Here's how the part is built. I have some questions about the finished solid (model axes, mm). A direction names the side the tool comes from. Round coordinates to 2 decimals unless told otherwise and drop trailing zeros. Write each loop counter-clockwise with the first axis right and the second up, starting at its lowest first coordinate (ties: lowest second). Pieces come first, ordered by that corner, then holes. Notation, with made-up numbers: (29.5, -0.5) - (66.5, -0.5) arc R8 ccw to (66.5, 11.5) - close; hole circle Ø6 at (-2, 66). An arc over 180 degrees is marked (long way). Return JSON: item names as keys, results as strings. Group by question number.
```python
from build123d import *

# Parameters (mm, degrees)
F0_W     = 48.26
F0_H     = 23.622
F1_DEPTH = 1.5875
F2_R     = 2.794
F2_R_2   = 1.016
F3_DEPTH = 3.175
F4_DEPTH = 6.35
F5_W     = 7.62
F5_H     = 12.7
F6_DEPTH = 6.35


with BuildPart() as f1:
    # F0 (on Top) → F1 (new body)
    with BuildSketch(Plane.XY):
        Rectangle(F0_W, F0_H)
    extrude(amount=F1_DEPTH)

    # F2 (on face) → F3 (join)
    with BuildSketch(Plane.XY.offset(1.5875)):
        with Locations((-17.018, 8.509)):
            Circle(F2_R)
        with Locations((-17.018, 8.509)):
            Circle(F2_R_2, mode=Mode.SUBTRACT)
        with Locations((17.018, -9.017)):
            Circle(F2_R)
        with Locations((17.018, -9.017)):
            Circle(F2_R_2, mode=Mode.SUBTRACT)
        with BuildLine():
            ThreePointArc((17.018, -11.811), (18.993656, -10.992656), (19.812, -9.017))
            ThreePointArc((19.812, -9.017), (15.042344, -7.041344), (17.018, -11.811))
        make_face()
        with Locations((17.018, -9.017)):
            Circle(F2_R_2, mode=Mode.SUBTRACT)
    extrude(amount=F3_DEPTH)

    # F2 (on face) → F4 (cut)
    with BuildSketch(Plane.XY.offset(1.5875)):
        with Locations((-17.018, 8.509)):
            Circle(F2_R_2)
        with Locations((17.018, -9.017)):
            Circle(F2_R_2)
    extrude(amount=-F4_DEPTH, mode=Mode.SUBTRACT)

    # F5 (on face) → F6 (cut)
    with BuildSketch(Plane.XY.offset(1.5875)):
        Polygon((-12.7, -9.525), (12.7, -9.525), (12.7, -3.175), (12.7, 9.525), (-12.7, 9.525), (-12.7, 3.175), align=None)
        with Locations((16.51, 3.175)):
            Rectangle(F5_W, F5_H)
        with Locations((-16.51, -3.175)):
            Rectangle(F5_W, F5_H)
    extrude(amount=-F6_DEPTH, mode=Mode.SUBTRACT)


solid = f1.part
```
1) Imagine slicing it at B-B (y = 2.5). Please give me the cut outline in (x, z), plus the area to 3 significant figures.
2) Imagine slicing it at A-A (x = -12). Please give me the cut outline in (y, z) (1 decimal).
3) I need wall thicknesses on line 1 along Y through (x, z) = (14, 0.8) (3 decimals); line 2 along X through (y, z) = (5.5, 0.2); line 3 along Y through (x, z) = (17, 1.25) (3 decimals). Which ranges of each line are inside material? Lowest first, please.
4) Will this pin go through, and if not, where does the flat tip stop? pin 1 Ø1.6 at (x, y) = (-17.018, 8.509) entering from +Z.
5) For faces 1 (the flat face through (0, -10, 0)), 2 (the cylindrical face through (14.54, -10.31, 3.15)), 3 (the flat face through (12.7, -6, 1)), which set-ups out of +Z, -Z, +X, -X, +Y, -Y let a thin tool reach every point of the face, with its end or its side?
6) Imagine slicing it at D-D (z = 3.15). Please give me the cut outline in (x, y), plus the area to 3 significant figures.
7) If we mould it in two halves opening along X, with no side actions, what happens to faces 4 (the cylindrical face through (-19.235, 6.809, 3.153)), 5 (the flat face through (-20.32, -3, 1)), 6 (the flat face through (0, -10, 1.588))? For each: released by +X, released by -X, zero draft, split by the parting line, or undercut.
8) Imagine slicing it at C-C (z = 0.75). Please give me the cut outline in (x, y) (3 decimals), plus the area to 3 significant figures.
Results found:
{
 "1": {"outline": "(-24.13, 0) - (-20.32, 0) - (-20.32, 1.59) - (-24.13, 1.59) - close; (20.32, 0) - (24.13, 0) - (24.13, 1.59) - (20.32, 1.59) - close", "area": "12.1 mm²"},
 "2": {"outline": "(-11.8, 0) - (-9.5, 0) - (-9.5, 1.6) - (-11.8, 1.6) - close; (9.5, 0) - (11.8, 0) - (11.8, 1.6) - (9.5, 1.6) - close"},
 "3": {"line 1": "y = -11.811 to -3.175, 9.525 to 11.811", "line 2": "x = -24.13 to -12.7, 20.32 to 24.13", "line 3": "y = -11.811 to -10.033, -8.001 to -3.175, 9.525 to 11.811"},
 "4": {"pin 1": "passes through"},
 "5": {"face 1": "-Z, +X, -X, +Y, -Y", "face 2": "+Z", "face 3": "+Z, -Z"},
 "6": {"outline": "circle Ø5.59 at (-17.02, 8.51); circle Ø5.59 at (17.02, -9.02); hole circle Ø2.03 at (-17.02, 8.51); hole circle Ø2.03 at (17.02, -9.02)", "area": "42.6 mm²"},
 "7": {"face 4": "split by the parting line", "face 5": "undercut", "face 6": "zero draft"},
 "8": {"outline": "(-24.13, -11.811) - (24.13, -11.811) - (24.13, 11.811) - (-24.13, 11.811) - close; hole (-20.32, -9.525) - (12.7, -9.525) - (12.7, -3.175) - (20.32, -3.175) - (20.32, 9.525) - (-12.7, 9.525) - (-12.7, 3.175) - (-20.32, 3.175) - close; hole circle Ø2.032 at (-17.018, 8.509); hole circle Ø2.032 at (17.018, -9.017)", "area": "456 mm²"}
}
